from build123d import *

# Parameters (mm, degrees)
F1_DEPTH     = 125
F2_DEPTH     = 10
F4_DEPTH     = 9.5
F5_T4_DEPTH  = 67.5870629671
F5_T9_DEPTH  = 55.4775446264
F5_T14_DEPTH = 67.5870629671
F5_T19_DEPTH = 63.0395446265


# Not quite as in the source:
# - a fillet or chamfer that OpenCascade refuses, or shapes differently, is made with other operations: its cross-section is extruded or revolved along the edge and cut away or added
# - a feature names something its author has since deleted; it is built from what else it names


with BuildPart() as f1:
    # F0 (on Top) → F1 (new body)
    with BuildSketch(Plane.XY):
        Polygon((-38.5, -38), (-38.5, -48), (38.5, -48), (38.5, -38), (5, -10), (10, 10), (38.5000000008, 38), (38.5, 48), (-38.5, 48), (-38.5000000011, 38), (-10, 10), (-5, -10), align=None)
        Polygon((-0.5119467155, -11.462), (0.5119467155, -11.462), (34.5, -39.8699251333), (34.5, -44), (-34.5, -44), (-34.5, -39.8699251333), align=None, mode=Mode.SUBTRACT)
        Polygon((-5.5209720151, 8.1640000003), (5.5209720151, 8.1640000003), (1.739972015, -6.96), (-1.739972015, -6.96), align=None, mode=Mode.SUBTRACT)
        Polygon((34.5000000007, 39.6776277195), (6.3932717857, 12.0640000003), (-6.3932717857, 12.0640000003), (-34.5000000007, 39.6776277195), (-34.5000000005, 44), (34.5000000003, 44), align=None, mode=Mode.SUBTRACT)
        Polygon((1.739972015, -6.96), (5.5209720151, 8.1640000003), (-5.5209720151, 8.1640000003), (-1.739972015, -6.96), align=None)
    extrude(amount=F1_DEPTH)

    # F0 (on Top) → F2 (cut)
    with BuildSketch(Plane.XY):
        Polygon((1.739972015, -6.96), (5.5209720151, 8.1640000003), (-5.5209720151, 8.1640000003), (-1.739972015, -6.96), align=None)
    extrude(amount=F2_DEPTH, mode=Mode.SUBTRACT)

    # F3 (on face) → F4 (join)
    with BuildSketch(Plane.XY.offset(125)):
        Polygon((1.739972015, -6.96), (5.5209720151, 8.1640000003), (-5.5209720151, 8.1640000003), (-1.739972015, -6.96), align=None)
    extrude(amount=F4_DEPTH)

    # F5: chamfer of 10 x 0.5 on 4 edges, made by hand


with BuildPart() as f5_tool2:
    # F5_s3 → F5_t4 (new body)
    with BuildSketch(Plane(origin=(-7.8409310443, -31.3637241773, 0), x_dir=(0, 0, 1), z_dir=(0.242535625, 0.9701425001, 0))):
        Polygon((124.5, 3.3760687511), (134.5, 2.8760687511), (134.5, 3.3760687511), align=None)
    extrude(amount=F5_T4_DEPTH)

    split(bisect_by=Plane.XY.offset(125), keep=Keep.TOP)


with BuildPart() as f1_1:
    add(f1.part)

    # F5_t1: cut F5_tool2
    add(f5_tool2.part, mode=Mode.SUBTRACT)


with BuildPart() as f5_tool7:
    # F5_s8 → F5_t9 (new body)
    with BuildSketch(Plane.YZ.offset(-27.7387723132)):
        Polygon((-6.96, 124.5), (-6.46, 134.5), (-6.96, 134.5), align=None)
    extrude(amount=F5_T9_DEPTH)

    split(bisect_by=Plane.XY.offset(125), keep=Keep.TOP)


with BuildPart() as f1_2:
    add(f1_1.part)

    # F5_t6: cut F5_tool7
    add(f5_tool7.part, mode=Mode.SUBTRACT)


with BuildPart() as f5_tool12:
    # F5_s13 → F5_t14 (new body)
    with BuildSketch(Plane(origin=(-8.5513395168, 34.2053580671, 0), x_dir=(0, 0, 1), z_dir=(0.242535625, -0.9701425001, 0))):
        Polygon((124.5, 3.3760687511), (134.5, 2.8760687511), (134.5, 3.3760687511), align=None)
    extrude(amount=F5_T14_DEPTH)

    split(bisect_by=Plane.XY.offset(125), keep=Keep.TOP)


with BuildPart() as f1_3:
    add(f1_2.part)

    # F5_t11: cut F5_tool12
    add(f5_tool12.part, mode=Mode.SUBTRACT)


with BuildPart() as f5_tool17:
    # F5_s18 → F5_t19 (new body)
    with BuildSketch(Plane.YZ.offset(31.5197723133)):
        Polygon((8.1640000003, 124.5), (7.6640000003, 134.5), (8.1640000003, 134.5), align=None)
    extrude(amount=-F5_T19_DEPTH)

    split(bisect_by=Plane.XY.offset(125), keep=Keep.TOP)


with BuildPart() as f1_4:
    add(f1_3.part)

    # F5_t16: cut F5_tool17
    add(f5_tool17.part, mode=Mode.SUBTRACT)


solid = f1_4.part
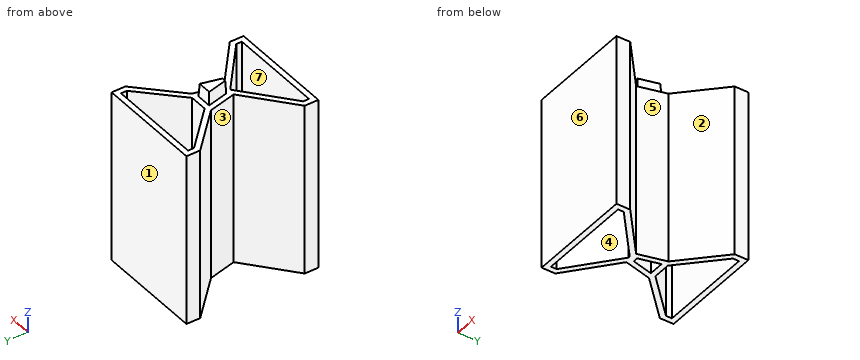
Part model, mm, in its own coordinate system. Face numbers are marked on the shaded views. A direction names the side the tool comes from. Coordinates: 2 decimals unless noted, no trailing zeros. Loops run counter-clockwise (first coordinate to the right, second up) from the corner with the lowest first, then second, coordinate; pieces in that order, holes last. Notation, with made-up numbers: (11, -24) - (49, -24) arc R24 ccw to (49, -1) - close; hole circle Ø10 at (-25, 70.5). An arc over 180 degrees is marked (long way). Write each question's results on one line, items separated by ' | '. Start each with the question number.
Q1. Probe line 1 along Y through (x, z) = (-32, 82); line 2 along Y through (x, z) = (-4, 25); line 3 along Y through (x, z) = (26, 77). List the from-to ranges inside material, lowest first.
Q2. Slice it at D-D on x = -33. Give the cut face in (y, z).
Q3. Slice it at C-C on z = 14. Give the cut face in (x, y).
Q4. Which spindle directions (+Z, -Z, +X, -X, +Y, -Y) get a long thin tool onto all of the face, cutting with end or side? Do the marked faces 1, 2, 3 and 4. Say none if no direction does.
Q5. Slice it at A-A on x = -8.5. Give the cut face in (y, z), and give its area (3 significant figures).
Q6. Two-plate mould, pull along X, no slides. Class the marked faces 5, 6 and 7: +X half, -X half, draft (parallel to the pull), parting line (faces both ways), or undercut.
Q7. Slice it at B-B on y = 21.5. Give the cut face in (x, z).
Q8. Drop flat-ended pins along their axis: pin 1 Ø1 at (y, z) = (-36.5, 38.5) entering from -X; pin 2 Ø6 at (y, z) = (-31.5, 30) entering from +X; pin 3 Ø1.5 at (x, y) = (-2.5, 11) entering from +Z. Give the stop position or say it passes through.
Answer:
1) line 1: y = -48 to -44, -37.78 to -32.57, 31.61 to 37.22, 44 to 48 | line 2: y = -48 to -44, -14.38 to 12.06, 44 to 48 | line 3: y = -48 to -44, -32.77 to -27.55, 25.72 to 31.33, 44 to 48
2) outline: (-48, 0) - (-44, 0) - (-44, 125) - (-48, 125) - close; (-38.62, 0) - (-33.4, 0) - (-33.4, 125) - (-38.62, 125) - close; (32.6, 0) - (38.2, 0) - (38.2, 125) - (32.6, 125) - close; (44, 0) - (48, 0) - (48, 125) - (44, 125) - close
3) outline: (-38.5, -48) - (38.5, -48) - (38.5, -38) - (5, -10) - (10, 10) - (38.5, 38) - (38.5, 48) - (-38.5, 48) - (-38.5, 38) - (-10, 10) - (-5, -10) - (-38.5, -38) - close; hole (-34.5, -44) - (34.5, -44) - (34.5, -39.87) - (0.51, -11.46) - (-0.51, -11.46) - (-34.5, -39.87) - close; hole (-34.5, 39.68) - (-6.39, 12.06) - (6.39, 12.06) - (34.5, 39.68) - (34.5, 44) - (-34.5, 44) - close
4) face 1: +Z, -Z, +X, -X, +Y | face 2: +Z, -Z, +X | face 3: +Z, -Z, -X | face 4: +Z, -Z
5) outline: (-48, 0) - (-44, 0) - (-44, 125) - (-48, 125) - close; (-18.14, 0) - (-12.93, 0) - (-12.93, 125) - (-18.14, 125) - close; (4, 0) - (14.13, 0) - (14.13, 125) - (4, 125) - close; (44, 0) - (48, 0) - (48, 125) - (44, 125) - close | area: 2,920 mm2
6) face 5: +X half | face 6: draft | face 7: undercut
7) outline: (-21.71, 0) - (-16, 0) - (-16, 125) - (-21.71, 125) - close; (16, 0) - (21.71, 0) - (21.71, 125) - (16, 125) - close
8) pin 1: stops at x = -37.3 | pin 2: stops at x = 34.31 | pin 3: stops at z = 125
